Design review of the part built by this model. Coordinates are the model's own, in mm. Give positions to 0.01 mm unless a question says otherwise; leave off trailing zeros. Write each loop counter-clockwise with the first axis right and the second up, starting at its lowest first coordinate (ties: lowest second). Pieces come first, ordered by that corner, then holes. Notation, with made-up numbers: M 21,79 L 57,79 A33 ccw 57,110 Z; hole C 81,-25 d4. An arc over 180 degrees is marked long. Write each question's results on one line, items separated by ' | '. Start each with the question number.
from build123d import *

# Parameters (mm, degrees)
SKETCH1_R                                           = 4
BOSS_EXTRUDE1_DEPTH                                 = 10
CSK_FOR_1_4_FLAT_HEAD_MACHINE_SCREW_100_D           = 7.14248
CSK_FOR_1_4_FLAT_HEAD_MACHINE_SCREW_100_CSINK_D     = 12.8778
CSK_FOR_1_4_FLAT_HEAD_MACHINE_SCREW_100_CSINK_ANGLE = 100


with BuildPart() as part:
    # Sketch1 → Boss-Extrude1 (new body)
    with BuildSketch(Plane(origin=(0, 0, 0), x_dir=(1, 0, 0), z_dir=(0, 1, 0))):
        with BuildLine():
            Line((-62.460834708, 11.244058758), (-63.909867943, 8.573388842))
            Line((-63.909867943, 8.573388842), (-63.829432577, 5.536004231))
            ThreePointArc((-63.829432577, 5.536004231), (-63.097972523, 4.842285457), (-63.791691298, 4.110825404))
            Line((-63.791691298, 4.110825404), (-63.711255932, 1.073440793))
            Line((-63.711255932, 1.073440793), (-62.122904556, -1.516793758))
            ThreePointArc((-62.122904556, -1.516793758), (-61.142582181, -1.751841812), (-61.377630236, -2.732164188))
            Line((-61.377630236, -2.732164188), (-59.78927886, -5.322398739))
            Line((-59.78927886, -5.322398739), (-57.118608944, -6.771431974))
            ThreePointArc((-57.118608944, -6.771431974), (-56.152100835, -6.484828372), (-55.865497234, -7.451336481))
            Line((-55.865497234, -7.451336481), (-53.194827318, -8.900369716))
            Line((-53.194827318, -8.900369716), (-50.157442707, -8.81993435))
            ThreePointArc((-50.157442707, -8.81993435), (-49.463723933, -8.088474296), (-48.732263879, -8.782193071))
            Line((-48.732263879, -8.782193071), (-45.694879269, -8.701757705))
            Line((-45.694879269, -8.701757705), (-43.104644718, -7.11340633))
            ThreePointArc((-43.104644718, -7.11340633), (-42.869596663, -6.133083954), (-41.889274288, -6.368132009))
            Line((-41.889274288, -6.368132009), (-39.299039737, -4.779780634))
            Line((-39.299039737, -4.779780634), (-37.850006502, -2.109110717))
            ThreePointArc((-37.850006502, -2.109110717), (-38.136610103, -1.142602609), (-37.170101995, -0.855999007))
            Line((-37.170101995, -0.855999007), (-35.72106876, 1.814670909))
            Line((-35.72106876, 1.814670909), (-35.801504126, 4.852055519))
            ThreePointArc((-35.801504126, 4.852055519), (-36.532964179, 5.545774294), (-35.839245405, 6.277234347))
            Line((-35.839245405, 6.277234347), (-35.919680771, 9.314618958))
            Line((-35.919680771, 9.314618958), (-37.508032146, 11.904853509))
            ThreePointArc((-37.508032146, 11.904853509), (-38.488354522, 12.139901563), (-38.253306467, 13.120223939))
            Line((-38.253306467, 13.120223939), (-39.841657842, 15.71045849))
            Line((-39.841657842, 15.71045849), (-42.512327759, 17.159491725))
            ThreePointArc((-42.512327759, 17.159491725), (-43.478835867, 16.872888123), (-43.765439468, 17.839396232))
            Line((-43.765439468, 17.839396232), (-46.436109385, 19.288429467))
            Line((-46.436109385, 19.288429467), (-49.473493995, 19.207994101))
            ThreePointArc((-49.473493995, 19.207994101), (-50.16721277, 18.476534047), (-50.898672823, 19.170252822))
            Line((-50.898672823, 19.170252822), (-53.936057434, 19.089817456))
            Line((-53.936057434, 19.089817456), (-56.526291984, 17.501466081))
            ThreePointArc((-56.526291984, 17.501466081), (-56.761340039, 16.521143705), (-57.741662415, 16.75619176))
            Line((-57.741662415, 16.75619176), (-60.331896965, 15.167840385))
            Line((-60.331896965, 15.167840385), (-61.7809302, 12.497170468))
            ThreePointArc((-61.7809302, 12.497170468), (-61.494326599, 11.530662359), (-62.460834708, 11.244058758))
        make_face()
        with Locations(Location((-49.815468351, 5.194029875, 0), (0, 0, 270))):
            Circle(SKETCH1_R, mode=Mode.SUBTRACT)
    extrude(amount=BOSS_EXTRUDE1_DEPTH)

    # CSK for 1/4 Flat Head Machine Screw (100)1 (through all)
    with Locations(Plane(origin=(-49.815468351, 10, -5.194029875), x_dir=(0, 0, 1), z_dir=(0, 1, 0))):
        with Locations((0, 0)):
            CounterSinkHole(CSK_FOR_1_4_FLAT_HEAD_MACHINE_SCREW_100_D / 2, CSK_FOR_1_4_FLAT_HEAD_MACHINE_SCREW_100_CSINK_D / 2, counter_sink_angle=CSK_FOR_1_4_FLAT_HEAD_MACHINE_SCREW_100_CSINK_ANGLE)


solid = part.part
Q1. We need section B-B on x = -40.75. Write out the cut boundary in (y, z).
Q2. For pin 1 Ø3 at (y, z) = (6, -15) entering from -X; pin 2 Ø4 at (y, z) = (5.5, -8) entering from +X, all flat-tipped, find the tip position at first contact; note any pin that passes through.
Q3. We need section A-A on z = 3.5. Write out the cut boundary in (x, y), and give its area (3 significant figures).
Q4. The part is to be moulded in two halves that separate along Z. For faces 1 (the flat face through (-63.175, 4.93, -9.927)), 2 (the conical face through (-46.343, 8.053, -7.408)), 3 (the flat face through (-54.549, 4.93, 8.166)), say which applies: pulls with the +Z half, pulls with the -Z half, needs draft (parallel to the pull), parting line crosses it, or undercut.
Q5. Wall thickness on line 1 along Z through (x, y) = (-52, 0.5); line 2 along X through (y, z) = (3.75, -5); line 3 along X through (y, z) = (6.5, -7.25) (3 decimals): over which ranges is each line inside the solid? List them lowest first. Write a range as from..to.
Answer sheet:
1) outline: M 0,-16.2 L 10,-16.2 L 10,5.67 L 0,5.67 Z
2) pin 1: x = -61.24 | pin 2: x = -35.84
3) outline: M -60.91,0 L -38.6,0 L -38.6,10 L -60.91,10 Z | area: 223 mm^2
4) face 1: pulls with the -Z half | face 2: undercut | face 3: pulls with the +Z half
5) line 1: -19.14..-8.54, -1.84..8.87 | line 2: -63.12..-53.81, -45.82..-36.26 | line 3: -63.875..-53.247, -46.384..-35.865
